Verification items for this drawing (mm, ordinates from the low corner). Coordinates: 2 decimals unless noted, no trailing zeros. Loops run counter-clockwise (first coordinate to the right, second up) from the corner with the lowest first, then second, coordinate; pieces in that order, holes last. Notation, with made-up numbers: (41.5, -24) -> (96.5, -24) arc R33 ccw to (96.5, 6) -> close; hole circle Ø7 at (-27, 61). An arc over 180 degrees is marked (long way). Write item = value, one per line.
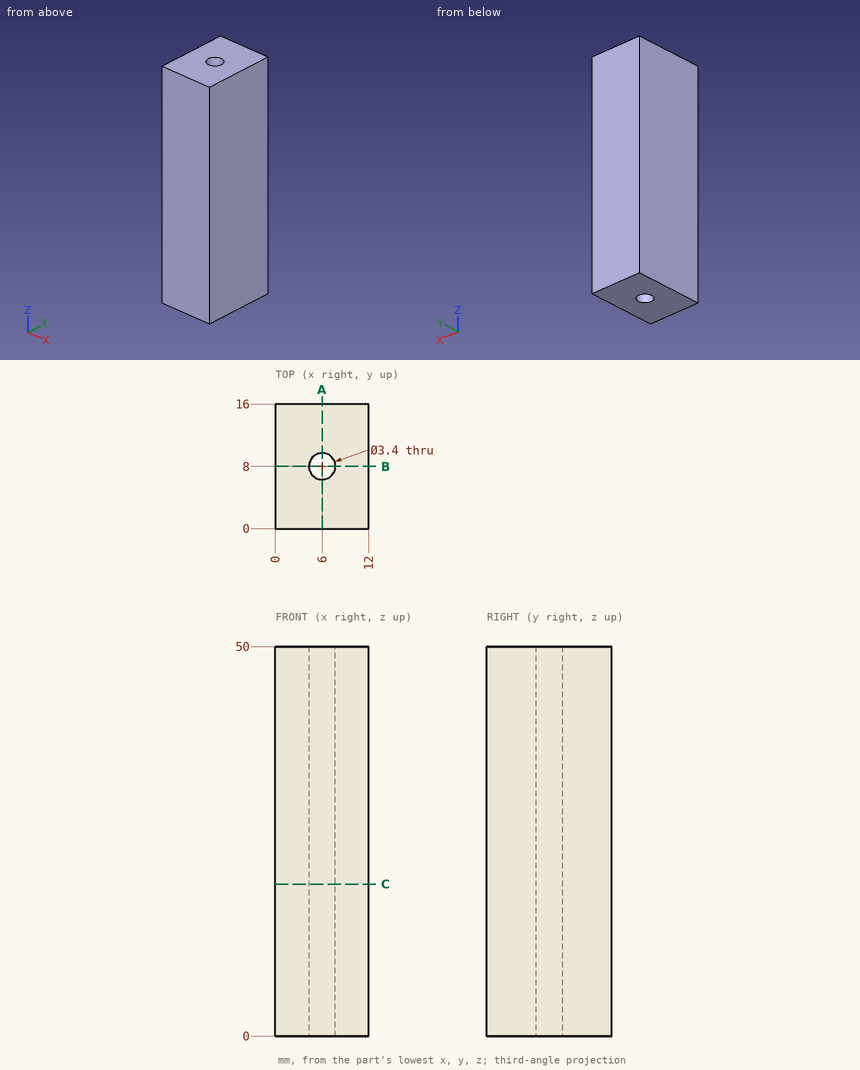
1) Sectioned sample at A-A, the plane x = 6. Record the cut outline in (y, z), plus the area to 3 significant figures.
Ans:
outline = (0, 0) -> (6.3, 0) -> (6.3, 50) -> (0, 50) -> close; (9.7, 0) -> (16, 0) -> (16, 50) -> (9.7, 50) -> close
area = 630 mm2
2) Material ranges on line 1 (Y direction, x = 6, z = 15.5); line 2 (X direction, y = 6.75, z = 47.5); line 3 (Y direction, x = 6.5, z = 7), recorded low to high.
Ans:
line_1 = 0 to 6.3, 9.7 to 16
line_2 = 0 to 4.85, 7.15 to 12
line_3 = 0 to 6.38, 9.62 to 16
3) Sectioned sample at C-C, the plane z = 19.5. Record the cut outline in (x, y), plus the area to 3 significant figures.
Ans:
outline = (0, 0) -> (12, 0) -> (12, 16) -> (0, 16) -> close; hole circle Ø3.4 at (6, 8)
area = 183 mm2
4) Sectioned sample at B-B, the plane y = 8. Record the cut outline in (x, z).
Ans:
outline = (0, 0) -> (4.3, 0) -> (4.3, 50) -> (0, 50) -> close; (7.7, 0) -> (12, 0) -> (12, 50) -> (7.7, 50) -> close
